from build123d import *

# Parameters (mm, degrees)
SKETCH1_R                        = 7.9375
SKETCH1_R_2                      = 3.3782
BOSS_EXTRUDE1_DEPTH              = 3.175
F_10_0_1935_DIAMETER_HOLE1_D     = 4.9149
F_1_4_0_25_DIAMETER_HOLE2_D      = 6.35
F_10_0_1935_DIAMETER_HOLE2_D     = 4.9149
F_10_0_1935_DIAMETER_HOLE2_DEPTH = 12.0396
F_10_0_1935_DIAMETER_HOLE2_TIP   = 1.476584928


with BuildPart() as part:
    # Sketch1 → Boss-Extrude1 (new body)
    with BuildSketch(Plane(origin=(0, 0, 0), x_dir=(1, 0, 0), z_dir=(0, 1, 0))):
        with BuildLine():
            ThreePointArc((21.773129464, 18.505714208), (-22.309015306, 17.856048305), (-13.287106438, -25.297893737))
            ThreePointArc((-13.287106438, -25.297893737), (44.264595617, -34.002230789), (94.865631565, -5.235947505))
            ThreePointArc((94.865631565, -5.235947505), (95.083258514, 4.977069459), (85.059583132, 6.946589417))
            ThreePointArc((85.059583132, 6.946589417), (51.353410938, 1.431482164), (21.773129464, 18.505714208))
        make_face()
        Circle(SKETCH1_R, mode=Mode.SUBTRACT)
        with Locations((88.9, 0)):
            Circle(SKETCH1_R_2, mode=Mode.SUBTRACT)
    extrude(amount=BOSS_EXTRUDE1_DEPTH)

    # #10 (0.1935) Diameter Hole1 (through all)
    with Locations(Plane(origin=(0, 3.175, 0), x_dir=(1, 0, 0), z_dir=(0, 1, 0))):
        with Locations((0, -23.8125), (-20.622229928, 11.90625), (20.622229928, 11.90625), (20.622229928, -11.90625), (-20.622229928, -11.90625), (0, 23.8125)):
            Hole(F_10_0_1935_DIAMETER_HOLE1_D / 2)

    # 1/4 (0.25) Diameter Hole2 (through all)
    with Locations(Plane(origin=(0, 3.175, 0), x_dir=(1, 0, 0), z_dir=(0, 1, 0))):
        with Locations((38.1, -7.9375)):
            Hole(F_1_4_0_25_DIAMETER_HOLE2_D / 2)

    # #10 (0.1935) Diameter Hole2
    with Locations(Plane(origin=(0, 3.175, 0), x_dir=(1, 0, 0), z_dir=(0, 1, 0))):
        with Locations((68.58, -8.680112147), (45.72, -18.445238312)):
            Hole(F_10_0_1935_DIAMETER_HOLE2_D / 2, depth=F_10_0_1935_DIAMETER_HOLE2_DEPTH)
            with Locations((0, 0, -(F_10_0_1935_DIAMETER_HOLE2_DEPTH + F_10_0_1935_DIAMETER_HOLE2_TIP / 2))):  # 118° drill point
                Cone(0, F_10_0_1935_DIAMETER_HOLE2_D / 2, F_10_0_1935_DIAMETER_HOLE2_TIP, mode=Mode.SUBTRACT)


solid = part.part
Model file for the job. Use its own axes, mm. Give positions to 0.01 mm unless a question says otherwise; leave off trailing zeros. Loops run counter-clockwise (first coordinate to the right, second up) from the corner with the lowest first, then second, coordinate; pieces in that order, holes last.
1) Saw through at B-B (x = 38.1). Write the cut outline in (y, z) (1 decimal), plus the area to 3 significant figures.
2) Saw through at D-D (x = 69.5). Write the cut outline in (y, z) (3 decimals).
3) Pull direction X, two halves, no side cores. Call faces 1 (the cylindrical face through (43.45, 1.57, 19.39)), 2 (the flat face through (19, 0, 3)), 3 (the cylindrical face through (-21.86, 1.57, -18.4)): +X half, -X half, draft (parallel to the pull), parting line (faces both ways), or undercut.
4) Wall check: line 1 (X direction, y = 2.7, z = 13.5); line 2 (X direction, y = 0.6, z = -5); line 3 (X direction, y = 0.8, z = -23). Give the ranges that are in metal, low to high.
5) Flat gauge pins, fed straight in: pin 1 Ø1 at (y, z) = (2.5, -21.5) entering from -X; pin 2 Ø1 at (x, y) = (79.5, 2) entering from -Z; pin 3 Ø1.5 at (x, y) = (58.5, 2.5) entering from -Z. Where does each tip first touch, or does it go through?
6) Saw through at A-A (x = 0.5). Write the cut outline in (y, z) (3 decimals), plus the area to 3 significant figures.
7) Saw through at C-C (y = 1.3). Count the separate pieces of the cut face and the enclosed holes in it, plus the area to 3 significant figures.
Answer block:
1. outline: (0, -5.8) - (3.2, -5.8) - (3.2, 4.8) - (0, 4.8) - close; (0, 11.1) - (3.2, 11.1) - (3.2, 34.9) - (0, 34.9) - close
1. area: 109 mm2
2. outline: (0, -1.412) - (3.175, -1.412) - (3.175, 6.401) - (0, 6.401) - close; (0, 10.959) - (3.175, 10.959) - (3.175, 25.239) - (0, 25.239) - close
3. face 1: undercut
3. face 2: draft
3. face 3: parting line
4. line 1: x = -25.18 to -22.49, -18.75 to 18.75, 22.49 to 86.59
4. line 2: x = -28.13 to -6.16, 6.16 to 39.81, 81.15 to 95.06
4. line 3: x = -16.96 to -2.32, 2.32 to 16.96
5. pin 1: stops at x = -19.38
5. pin 2: stops at z = -4.5
5. pin 3: stops at z = -0.68
6. outline: (0, -28.571) - (3.175, -28.571) - (3.175, -26.219) - (0, -26.219) - close; (0, -21.406) - (3.175, -21.406) - (3.175, -7.922) - (0, -7.922) - close; (0, 7.922) - (3.175, 7.922) - (3.175, 21.406) - (0, 21.406) - close; (0, 26.219) - (3.175, 26.219) - (3.175, 31.117) - (0, 31.117) - close
6. area: 109 mm2
7. separate pieces: 1
7. enclosed holes: 11
7. area: 4,520 mm2
